Autodesk Inventor part; units mm, degrees
ref_plane "YZ Plane" through (0, 0, 0) normal (1, 0, 0) x (0, 1, 0)
ref_plane "XZ Plane" through (0, 0, 0) normal (0, 1, 0) x (-1, 0, 0)
ref_plane "XY Plane" through (0, 0, 0) normal (0, 0, 1) x (1, 0, 0)
sketch "Sketch1" plane through (0, 0, 0) normal (0, 1, 0) x (-1, 0, 0)
  circle A0 centre (0, 0) radius 16.575
  circle A1 centre (0, 0) radius 2.5
  dimension "d0" = 33.15
  dimension "d1" = 5
extrude "Extrusion1" add sketch "Sketch1" along normal blind 3.8
sketch "Sketch2" plane through (0, 3.8, 0) normal (0, 1, 0) x (1, 0, 0)
  circle A0 centre (0, 0) radius 2.5
  circle A1 centre (0, 0) radius 16.575
  line L0 (-2.5, 0) -> (-16.575, 0)
  circle A2 centre (-9.5375, 0) radius 1.5
  line L1 (0, 0) -> (16.575, 0) construction
  line L2 (0, 0) -> (16.575, 0) construction
  circle A3 centre (4.7688, 8.2597) radius 1.5
  circle A4 centre (4.7688, -8.2597) radius 1.5
  dimension "d4" = 3
  dimension "d7" = 3
  dimension "d8" = 3
extrude "Extrusion2" cut sketch "Sketch2" against normal blind 3.8 contours A2 L0 | L0 A2 | A3 | A4
sketch "Sketch3" plane through (0, 0, 0) normal (0, -1, 0) x (1, 0, 0)
  circle A0 centre (0, 0) radius 16.575
  circle A1 centre (0, 0) radius 17.325
  dimension "d11" = 34.65
extrude "Extrusion3" add sketch "Sketch3" against normal blind 3.8
sketch "Sketch4" plane through (0, 0, 0) normal (0, -1, 0) x (1, 0, 0)
  circle A0 centre (4.7688, -8.2597) radius 1.5
  circle A1 centre (-9.5375, 0) radius 1.5
  circle A2 centre (4.7688, 8.2597) radius 1.5
extrude "Extrusion4" add sketch "Sketch4" against normal blind 3.8
sketch "Sketch5" plane through (0, 0, 0) normal (0, -1, 0) x (1, 0, 0)
  circle A0 centre (0, 0) radius 17.325
  circle A1 centre (0, 0) radius 2.5
  line L0 (-2.5, 0) -> (-17.325, 0)
  circle A2 centre (-9.9125, 0) radius 1
  line L1 (0, 0) -> (17.325, 0) construction
  line L2 (0, 0) -> (17.325, 0) construction
  circle A3 centre (4.9563, -8.5845) radius 1
  circle A4 centre (4.9563, 8.5845) radius 1
  dimension "d16" = 2
  dimension "d19" = 2
  dimension "d20" = 2
extrude "Extrusion5" cut sketch "Sketch5" against normal blind 3.8 contours A2 L0 | L0 A2 | A3 | A4
sketch "Sketch7" plane through (0, 3.8, 0) normal (0, 1, 0) x (1, 0, 0)
  circle A0 centre (4.9563, 8.5845) radius 1
  circle A1 centre (-9.9125, 0) radius 1
  circle A2 centre (4.9563, -8.5845) radius 1
  circle A3 centre (0, 0) radius 17.325
  circle A4 centre (0, 0) radius 2.5
extrude "Extrusion6" add sketch "Sketch7" along normal blind 0.3
properties part number "kolecko_rameno(2)"
Could you check a few things on this model? Use its own coordinates, in mm. Coordinates: 2 decimals unless noted, no trailing zeros. Loops run counter-clockwise (first coordinate to the right, second up) from the corner with the lowest first, then second, coordinate; pieces in that order, holes last. Notation, with made-up numbers: M 77,85 L 128,85 A12 cw 128,103 Z; hole C -5.75,37 d11. An arc over 180 degrees is marked long. Put each result on its own line as item: value. Start each with the question number.
(1) Suppose I cut it at A-A on z = 0. Please give me the cut outline in (x, y) (1 decimal), then the cut area to 3 significant figures.
(2) Suppose I cut it at D-D on y = 2.2. Count the separate pieces of the cut face and the enclosed holes in it, then the cut area to 3 significant figures.
(3) Will these pins go through, and if not, where does the flat tip stop? P1, Ø2.5, axis at x = 4.96, z = 8.58, coming from the -Y side; P2, Ø1.5, axis at x = -8.5, y = 1, coming from the +Z side; P3, Ø1.2, axis at x = 4.96, z = -8.58, coming from the +Y side; P4, Ø2, axis at y = 1.5, z = -10, coming from the -X side.
(4) I need wall thicknesses on line 1 (X direction, y = 2.25, z = 0) (1 decimal); line 2 (Z direction, x = 4.5, y = 0.45); line 3 (X direction, y = 2.8, z = 2). Which ranges of each line are inside material? Lowest first, please. Write a range as from..to.
(5) Suppose I cut it at B-B on x = 0. Please give me the cut outline in (y, z) (3 decimals), then the cut area to 3 significant figures.
(6) Suppose I cut it at C-C on x = 4.5. Please give me the cut outline in (y, z).
Solutions:
1. outline: M -17.3,0 L -10.9,0 L -10.9,4.1 L -17.3,4.1 Z; M -8.9,0 L -2.5,0 L -2.5,4.1 L -8.9,4.1 Z; M 2.5,0 L 17.3,0 L 17.3,4.1 L 2.5,4.1 Z
1. area: 113 mm2
2. separate pieces: 1
2. enclosed holes: 4
2. area: 914 mm2
3. P1: stops at y = 0
3. P2: stops at z = 15.49
3. P3: passes through
3. P4: stops at x = -14.8
4. line 1: x = -17.3..-10.9, -8.9..-2.5, 2.5..17.3
4. line 2: z = -16.73..-9.47, -7.69..7.69, 9.47..16.73
4. line 3: x = -17.21..-1.5, 1.5..17.21
5. outline: M 0,-17.325 L 4.1,-17.325 L 4.1,-2.5 L 0,-2.5 Z; M 0,2.5 L 4.1,2.5 L 4.1,17.325 L 0,17.325 Z
5. area: 122 mm2
6. outline: M 0,-16.73 L 4.1,-16.73 L 4.1,-9.47 L 0,-9.47 Z; M 0,-7.69 L 4.1,-7.69 L 4.1,7.69 L 0,7.69 Z; M 0,9.47 L 4.1,9.47 L 4.1,16.73 L 0,16.73 Z
